Autodesk Fusion 360 part; units mm, degrees
sketch "Esquisse1" plane through (0, 0, 0) normal (0, 0, 1) x (1, 0, 0)
  line L0 (8, -16) -> (-8, -16)
  line L1 (-12, -12) -> (-12, 12)
  line L2 (-8, 16) -> (8, 16)
  line L3 (12, 12) -> (12, -12)
  line L4 (12, -16) -> (-12, 16) construction
  line L5 (-12, -16) -> (12, 16) construction
  circle A0 centre (-8, -4) radius 2.425
  circle A1 centre (8, -4) radius 2.425
  circle A2 centre (0, 8) radius 5
  arc A3 (-12, -12) -> (-8, -16) centre (-8, -12) ccw
  arc A4 (8, -16) -> (12, -12) centre (8, -12) ccw
  arc A5 (12, 12) -> (8, 16) centre (8, 12) ccw
  arc A6 (-8, 16) -> (-12, 12) centre (-8, 12) ccw
  dimension "d1" = 24
  dimension "d2" = 32
  dimension "d3" = 4.85
  dimension "d4" = 4.85
  dimension "d5" = 12
  dimension "d6" = 12
  dimension "d7" = 16
  dimension "d8" = 10
  dimension "d9" = 8
  dimension "d10" = 4
extrude "Extrusion1" add sketch "Esquisse1" against normal blind 8 contours L0 L1 L2 L3 A3 A4 A5 A6 | A2
extrude "Extrusion2" add sketch "Esquisse1" along normal blind 25.4 contours A2
fillet "Congé1" radius 0.5 16 edges at (0, -16, -8) (-10.8284, -14.8284, -8) (-12, 0, -8) (-10.8284, 14.8284, -8) (0, 16, -8) (10.8284, 14.8284, -8) (12, 0, -8) (10.8284, -14.8284, -8) (10.8284, -14.8284, 0) (0, -16, 0) (-10.8284, -14.8284, 0) (-12, 0, 0) (-10.8284, 14.8284, 0) (0, 16, 0) (10.8284, 14.8284, 0) (12, 0, 0)
fillet "Congé2" radius 1.5 1 edges at (-4.6616, 6.1919, 25.4)
equation "d6 = d5"
The model under review builds one solid part; all positions refer to its coordinate system, in mm. Round coordinates to 2 decimals unless told otherwise and drop trailing zeros. Loops run counter-clockwise (first coordinate to the right, second up) from the corner with the lowest first, then second, coordinate; pieces in that order, holes last.
1) Consider section B-B on y = 8. State the section outline as (x, z) points.
Values follow:
outline: (-12, -7.5) arc R0.5 ccw to (-11.5, -8) - (11.5, -8) arc R0.5 ccw to (12, -7.5) - (12, -0.5) arc R0.5 ccw to (11.5, 0) - (5, 0) - (5, 23.9) arc R1.5 ccw to (3.5, 25.4) - (-3.5, 25.4) arc R1.5 ccw to (-5, 23.9) - (-5, 0) - (-11.5, 0) arc R0.5 ccw to (-12, -0.5) - close
2) Consider section A-A on y = -4. State the section outline as (x, z) points (3 decimals), then the cut area to 3 significant figures.
Values follow:
outline: (-12, -7.5) arc R0.5 ccw to (-11.5, -8) - (-10.425, -8) - (-10.425, 0) - (-11.5, 0) arc R0.5 ccw to (-12, -0.5) - close; (-5.575, -8) - (5.575, -8) - (5.575, 0) - (-5.575, 0) - close; (10.425, -8) - (11.5, -8) arc R0.5 ccw to (12, -7.5) - (12, -0.5) arc R0.5 ccw to (11.5, 0) - (10.425, 0) - close
area: 114 mm2
3) Clearance check with flat-ended pins moving along their axes: P1, Ø8, axis at x = 8, y = -4, coming from the +Z side; P2, Ø1.5, axis at x = 7.5, z = 10, coming from the -Y side; P3, Ø4, axis at y = 3.5, z = 17, coming from the +X side. State where each tip first meets the part, or that it passes through.
Values follow:
P1: stops at z = 0
P2: passes through
P3: stops at x = 4.33
4) The part is to be moulded in two halves that separate along X. For faces 1 (the face through (5.577, -3.893, -3.944)), 2 (the face through (12, 0, -4)), 3 (the face through (-0.651, 3.043, 11.783)), say which applies: pulls with the +X half, pulls with the -X half, needs draft (parallel to the pull), parting line crosses it, or undercut.
Values follow:
face 1: undercut
face 2: pulls with the +X half
face 3: parting line crosses it
5) Consider section C-C on x = 0. State the section outline as (y, z) points, then the cut area to 3 significant figures.
Values follow:
outline: (-16, -7.5) arc R0.5 ccw to (-15.5, -8) - (15.5, -8) arc R0.5 ccw to (16, -7.5) - (16, -0.5) arc R0.5 ccw to (15.5, 0) - (13, 0) - (13, 23.9) arc R1.5 ccw to (11.5, 25.4) - (4.5, 25.4) arc R1.5 ccw to (3, 23.9) - (3, 0) - (-15.5, 0) arc R0.5 ccw to (-16, -0.5) - close
area: 509 mm2
6) Consider section D-D on x = -6. State the section outline as (y, z) points, then the cut area to 3 significant figures.
Values follow:
outline: (-16, -7.5) arc R0.5 ccw to (-15.5, -8) - (-5.37, -8) - (-5.37, 0) - (-15.5, 0) arc R0.5 ccw to (-16, -0.5) - close; (-2.63, -8) - (15.5, -8) arc R0.5 ccw to (16, -7.5) - (16, -0.5) arc R0.5 ccw to (15.5, 0) - (-2.63, 0) - close
area: 234 mm2
7) Wall thickness on line 1 along Y through (x, z) = (8, -2.5) (3 decimals); line 2 along Z through (x, y) = (10.5, -3); line 3 along Y through (x, z) = (10, -0.5): over which ranges is each line inside the solid? List them lowest first.
Values follow:
line 1: y = -16 to -6.425, -1.575 to 16
line 2: z = -8 to 0
line 3: y = -15.46 to -5.37, -2.63 to 15.46
